Could you check a few things on this model? Use its own coordinates, in mm. A direction names the side the tool comes from. Give positions to 0.01 mm unless a question says otherwise; leave off trailing zeros. Write each loop counter-clockwise with the first axis right and the second up, starting at its lowest first coordinate (ties: lowest second). Pieces come first, ordered by that corner, then holes. Notation, with made-up numbers: (79.25, 11.5) - (132.25, 11.5) arc R27 ccw to (132.25, 30.5) - close; hole circle Ø2 at (57.5, 39). An arc over 180 degrees is marked (long way). Use one line per item in the form item = value.
```python
from build123d import *

# Parameters (mm, degrees)
CROQUIS1_W              = 180
CROQUIS1_H              = 120
SALIENTE_EXTRUIR1_DEPTH = 7.9375


with BuildPart() as part:
    # Croquis1 → Saliente-Extruir1 (new body)
    with BuildSketch(Plane(origin=(0, 0, 0), x_dir=(1, 0, 0), z_dir=(0, 1, 0))):
        Rectangle(CROQUIS1_W, CROQUIS1_H)
        with BuildLine():
            Line((-65, -26), (65, -26))
            ThreePointArc((65, -26), (72.5, -33.5), (65, -41))
            Line((65, -41), (-65, -41))
            ThreePointArc((-65, -41), (-72.5, -33.5), (-65, -26))
        make_face(mode=Mode.SUBTRACT)
        with BuildLine():
            Line((-65, 41), (65, 41))
            ThreePointArc((65, 41), (72.5, 33.5), (65, 26))
            Line((65, 26), (-65, 26))
            ThreePointArc((-65, 26), (-72.5, 33.5), (-65, 41))
        make_face(mode=Mode.SUBTRACT)
    extrude(amount=SALIENTE_EXTRUIR1_DEPTH)


solid = part.part
```
1. If we mould it in two halves opening along X, with no side actions, what happens to faces 3 (the face through (-1, 7.938, -1)), 4 (the face through (-90, 4, 1)), 5 (the face through (-1, 4, -41))? For each: pulls with the +X half, pulls with the -X half, needs draft (parallel to the pull), parting line crosses it, or undercut.
Response values:
face_3 = needs draft
face_4 = pulls with the -X half
face_5 = undercut
2. Imagine slicing it at B-B, the plane x = 31.5. List the corners of the cut face in (y, z) for me, and give its area (3 significant figures).
Response values:
outline = (0, -60) - (7.94, -60) - (7.94, -41) - (0, -41) - close; (0, -26) - (7.94, -26) - (7.94, 26) - (0, 26) - close; (0, 41) - (7.94, 41) - (7.94, 60) - (0, 60) - close
area = 714 mm²
3. Imagine slicing it at C-C, the plane y = 2. List the corners of the cut face in (x, z) for me, and give its area (3 significant figures).
Response values:
outline = (-90, -60) - (90, -60) - (90, 60) - (-90, 60) - close; hole (-65, -41) - (65, -41) arc R7.5 ccw to (65, -26) - (-65, -26) arc R7.5 ccw to start; hole (-65, 26) - (65, 26) arc R7.5 ccw to (65, 41) - (-65, 41) arc R7.5 ccw to start
area = 17,300 mm²
4. Imagine slicing it at A-A, the plane z = -33.5. List the corners of the cut face in (x, y) for me.
Response values:
outline = (-90, 0) - (-72.5, 0) - (-72.5, 7.94) - (-90, 7.94) - close; (72.5, 0) - (90, 0) - (90, 7.94) - (72.5, 7.94) - close
5. If I drill on line 1 (Z direction, x = -38, y = 3.75); line 2 (Z direction, x = -66, y = 7.75); line 3 (X direction, y = 2.75, z = 36), over which ranges is the centre line in solid material (lowest first)? Write a range as from..to.
Response values:
line_1 = -60..-41, -26..26, 41..60
line_2 = -60..-40.93, -26.07..26.07, 40.93..60
line_3 = -90..-72.07, 72.07..90
6. Which directions (+Z, -Z, +X, -X, +Y, -Y) give clear straight access to the entire face, cutting with the end or side of a thin tool? Please do faces 1 (the face through (1, 4, -26)), 2 (the face through (-1, 4, 60)).
Response values:
face_1 = +Y, -Y
face_2 = +Z, +X, -X, +Y, -Y
